Geometry check sheet. Reference: the model listing, model coordinates, mm. A direction names the side the tool comes from. Give positions to 0.01 mm unless a question says otherwise; leave off trailing zeros. Loops run counter-clockwise (first coordinate to the right, second up) from the corner with the lowest first, then second, coordinate; pieces in that order, holes last.
```python
from build123d import *

# Parameters (mm, degrees)
SKETCH1_R           = 1.35
BOSS_EXTRUDE1_DEPTH = 3
FILLET1_R           = 5
FILLET2_R           = 1
BOSS_EXTRUDE2_DEPTH = 7
BOSS_EXTRUDE3_DEPTH = 1
CUT_EXTRUDE1_REACH  = 74.282
SKETCH3_R           = 3
CIRPATTERN3_COUNT   = 3


with BuildPart() as part:
    # Sketch1 → Boss-Extrude1 (new body)
    with BuildSketch(Plane(origin=(0, 0, 0), x_dir=(1, 0, 0), z_dir=(0, 1, 0))):
        with BuildLine():
            ThreePointArc((-18.950510257, 23.9), (-22.286742625, 24.785806775), (-24.760474821, 22.378370572))
            Line((-24.760474821, 22.378370572), (-28.023324698, 24.262177826))
            Line((-28.023324698, 24.262177826), (-35.023324698, 12.137822174))
            Line((-35.023324698, 12.137822174), (-23.9, 5.715767665))
            Line((-23.9, 5.715767665), (-23.9, -18.950510257))
            ThreePointArc((-23.9, -18.950510257), (-23.874873734, -23.874873734), (-18.950510257, -23.9))
            Line((-18.950510257, -23.9), (-7, -23.9))
            Line((-7, -23.9), (-7, -36.4))
            Line((-7, -36.4), (7, -36.4))
            Line((7, -36.4), (7, -23.9))
            Line((7, -23.9), (18.950510257, -23.9))
            ThreePointArc((18.950510257, -23.9), (23.874873734, -23.874873734), (23.9, -18.950510257))
            Line((23.9, -18.950510257), (23.9, 5.715767665))
            Line((23.9, 5.715767665), (35.023324698, 12.137822174))
            Line((35.023324698, 12.137822174), (28.023324698, 24.262177826))
            Line((28.023324698, 24.262177826), (24.760474821, 22.378370572))
            ThreePointArc((24.760474821, 22.378370572), (22.286742625, 24.785806775), (18.950510257, 23.9))
            Line((18.950510257, 23.9), (-18.950510257, 23.9))
        make_face()
        with Locations(Location((-21.4, -21.4, 0), (0, 0, 270))):
            Circle(SKETCH1_R, mode=Mode.SUBTRACT)
        Polygon((15.364466094, -18.9), (-15.364466094, -18.9), (0, -3.535533906), align=None, mode=Mode.SUBTRACT)
        with Locations(Location((21.4, -21.4, 0), (0, 0, 270))):
            Circle(SKETCH1_R, mode=Mode.SUBTRACT)
        Polygon((-3.535533906, 0), (-18.9, -15.364466094), (-18.9, 15.364466094), align=None, mode=Mode.SUBTRACT)
        with Locations(Location((-21.4, 21.4, 0), (0, 0, 270))):
            Circle(SKETCH1_R, mode=Mode.SUBTRACT)
        Polygon((18.9, -15.364466094), (3.535533906, 0), (18.9, 15.364466094), align=None, mode=Mode.SUBTRACT)
        Polygon((0, 3.535533906), (-15.364466094, 18.9), (15.364466094, 18.9), align=None, mode=Mode.SUBTRACT)
        with Locations(Location((21.4, 21.4, 0), (0, 0, 270))):
            Circle(SKETCH1_R, mode=Mode.SUBTRACT)
    extrude(amount=BOSS_EXTRUDE1_DEPTH)

    # Fillet1
    # the kernel refuses this fillet: 5 mm, written as the material it adds along each edge
    with BuildSketch(Plane(origin=(7, 0, 23.9), x_dir=(0, 0, 1), z_dir=(0, 1, 0)), Plane(origin=(-7, 0, 23.9), x_dir=(-1, 0, 0), z_dir=(0, 1, 0))) as fillet1_piece_1:
        with BuildLine():
            CenterArc((FILLET1_R, FILLET1_R), FILLET1_R, 180, 90)
            Line((0, FILLET1_R), (-FILLET1_R * 0.02, FILLET1_R))
            Line((-FILLET1_R * 0.02, FILLET1_R), (-FILLET1_R * 0.02, -FILLET1_R * 0.02))
            Line((-FILLET1_R * 0.02, -FILLET1_R * 0.02), (FILLET1_R, -FILLET1_R * 0.02))
            Line((FILLET1_R, -FILLET1_R * 0.02), (FILLET1_R, 0))
        make_face()
    extrude(amount=3)
    with BuildSketch(Plane(origin=(23.9, 0, 18.950510257), x_dir=(0.5912237553807399, 0, 0.8065075765753815), z_dir=(0, 1, 0)), Plane(origin=(-18.950510257, 0, 23.9), x_dir=(-0.806507576575308, 0, 0.5912237553808403), z_dir=(0, 1, 0)), Plane(origin=(18.950510257, 0, -23.9), x_dir=(0.8065075765752107, 0, -0.591223755380973), z_dir=(0, 1, 0))) as fillet1_piece_2:
        with BuildLine():
            CenterArc((1.705620507, 4.94923638), FILLET1_R, 233.756102233, 28.072486936)
            Line((-1.25049827, 0.916698497), (-1.309620646, 0.836047739))
            Line((-1.309620646, 0.836047739), (-0.059122376, -0.080650758))
            Line((-0.059122376, -0.080650758), (0.014213504, -0.098984728))
            ThreePointArc((0.014213504, -0.098984728), (0.497472648, -0.064465466), (0.980731791, -0.098984728))
            Line((0.980731791, -0.098984728), (0.994945296, 0))
        make_face()
    extrude(amount=3)
    with BuildSketch(Plane(origin=(18.950510257, 0, 23.9), x_dir=(-1, 0, 0), z_dir=(0, 1, 0)), Plane(origin=(-23.9, 0, 18.950510257), x_dir=(0, 0, -1), z_dir=(0, 1, 0)), Plane(origin=(-18.950510257, 0, -23.9), x_dir=(1, 0, 0), z_dir=(0, 1, 0))) as fillet1_piece_3:
        with BuildLine():
            CenterArc((1.550510257, 5), FILLET1_R, 241.927513064, 28.072486936)
            Line((-0.802430919, 0.588235294), (-0.849489743, 0.5))
            ThreePointArc((-0.849489743, 0.5), (-0.439328974, 0.24212576), (-0.069985421, -0.071428571))
            Line((-0.069985421, -0.071428571), (0, -0.1))
            Line((0, -0.1), (1.550510257, -0.1))
            Line((1.550510257, -0.1), (1.550510257, 0))
        make_face()
    extrude(amount=3)
    with BuildSketch(Plane(origin=(-23.9, 0, -5.715767665), x_dir=(-0.8660254037844421, 0, -0.49999999999999417), z_dir=(0, 1, 0)), Plane(origin=(23.9, 0, -5.715767665), x_dir=(0, 0, 1), z_dir=(0, 1, 0))) as fillet1_piece_4:
        with BuildLine():
            CenterArc((FILLET1_R * 0.57735026919, FILLET1_R), FILLET1_R, 210, 60)
            Line((-FILLET1_R * 0.288675134595, FILLET1_R * 0.5), (-FILLET1_R * 0.30599564267, FILLET1_R * 0.49))
            Line((-FILLET1_R * 0.30599564267, FILLET1_R * 0.49), (-FILLET1_R * 0.0115470053838, -FILLET1_R * 0.02))
            Line((-FILLET1_R * 0.0115470053838, -FILLET1_R * 0.02), (FILLET1_R * 0.57735026919, -FILLET1_R * 0.02))
            Line((FILLET1_R * 0.57735026919, -FILLET1_R * 0.02), (FILLET1_R * 0.57735026919, 0))
        make_face()
    extrude(amount=3)
    with BuildSketch(Plane(origin=(24.760474821, 0, -22.378370572), x_dir=(-0.6125107821213894, 0, -0.7904622329909531), z_dir=(0, 1, 0))) as fillet1_piece_5:
        with BuildLine():
            CenterArc((4.405584254, -4.650844222), FILLET1_R, 111.538849964, 57.883583887)
            Line((-0.509452241, -3.733011854), (-0.607752971, -3.714655207))
            ThreePointArc((-0.607752971, -3.714655207), (-0.353807697, -1.852984049), (-0.099081577, 0.013521878))
            Line((-0.099081577, 0.013521878), (0.036713202, 0.093016884))
            ThreePointArc((0.036713202, 0.093016884), (1.284962074, -0.144409045), (2.533210946, 0.093016884))
            Line((2.533210946, 0.093016884), (2.569924148, 0))
        make_face()
    extrude(amount=3)
    with BuildSketch(Plane(origin=(-24.760474821, 0, -22.378370572), x_dir=(0.6125107821216187, 0, -0.7904622329907753), z_dir=(0, 1, 0))) as fillet1_piece_6:
        with BuildLine():
            CenterArc((4.405584254, 4.650844222), FILLET1_R, 190.577566149, 57.883583887)
            Line((-0.509452241, 3.733011854), (-0.607752971, 3.714655207))
            ThreePointArc((-0.607752971, 3.714655207), (-0.353807697, 1.852984049), (-0.099081577, -0.013521878))
            Line((-0.099081577, -0.013521878), (0.036713202, -0.093016884))
            ThreePointArc((0.036713202, -0.093016884), (1.284962074, 0.144409045), (2.533210946, -0.093016884))
            Line((2.533210946, -0.093016884), (2.569924148, 0))
        make_face()
    extrude(amount=3)

    # Fillet2
    fillet2_edges = [part.edges().sort_by_distance(p)[0] for p in [
        (15.364466094, 1.5, -18.9),
        (-15.364466094, 1.5, -18.9),
        (0, 1.5, -3.535533906),
        (-18.9, 1.5, 15.364466094),
        (-3.535533906, 1.5, 0),
        (-18.9, 1.5, -15.364466094),
        (18.9, 1.5, 15.364466094),
        (18.9, 1.5, -15.364466094),
        (3.535533906, 1.5, 0),
        (-15.364466094, 1.5, 18.9),
        (15.364466094, 1.5, 18.9),
        (0, 1.5, 3.535533906),
    ]]
    fillet(fillet2_edges, radius=FILLET2_R)

    # Sketch2 → Boss-Extrude2 (add, symmetric)
    with BuildSketch(Plane(origin=(0, 0, 0), x_dir=(0, 0, -1), z_dir=(1, 0, 0))):
        Polygon((-36.4, 3), (-36.4, 0), (-38.701980964, 0), (-44.462888601, 21.5), (-59.462888601, 21.5), (-59.462888601, 23), (-41.758983849, 23), align=None)
    boss_extrude2 = extrude(amount=BOSS_EXTRUDE2_DEPTH, both=True)

    # Sketch2<3> → Boss-Extrude3 (add, symmetric)
    with BuildSketch(Plane(origin=(0, 0, 0), x_dir=(0, 0, -1), z_dir=(1, 0, 0))):
        Polygon((-33.294171459, 3), (-36.4, 3), (-41.758983849, 23), (-38.653155307, 23), align=None)
    boss_extrude3 = extrude(amount=BOSS_EXTRUDE3_DEPTH, both=True)

    # Sketch3 → Cut-Extrude1 (cut, up to next)
    with BuildSketch(Plane.XZ.offset(-21.5), mode=Mode.PRIVATE) as cut_extrude1_sk1:
        with Locations(Location((0, 52.462888601, 0), (0, 0, 270))):
            Circle(SKETCH3_R)
    cut_extrude1_tool1 = extrude(cut_extrude1_sk1.sketch, amount=-CUT_EXTRUDE1_REACH, mode=Mode.PRIVATE) & part.part
    cut_extrude1 = cut_extrude1_tool1.solids().sort_by_distance((0, 21.5, 52.462889))[0]
    add(cut_extrude1, mode=Mode.SUBTRACT)

    # CirPattern3: Boss-Extrude2, Boss-Extrude3, Cut-Extrude1 ×3 about axis
    cirpattern3_axis = Axis((0, 0, 0), (0, 1, 0))
    add([boss_extrude2.rotate(cirpattern3_axis, i * 360 / CIRPATTERN3_COUNT) for i in range(1, CIRPATTERN3_COUNT)])
    add([boss_extrude3.rotate(cirpattern3_axis, i * 360 / CIRPATTERN3_COUNT) for i in range(1, CIRPATTERN3_COUNT)])
    add([cut_extrude1.rotate(cirpattern3_axis, i * 360 / CIRPATTERN3_COUNT) for i in range(1, CIRPATTERN3_COUNT)], mode=Mode.SUBTRACT)


solid = part.part
```
1) Sectioned sample at B-B on z = 21.4. Enter the section's corners in (x, y).
2) Sectioned sample at C-C on y = 16. Enter the section's corners in (x, z).
3) Mould release check, pull along X, two halves, no side actions. Record for faces 1 (the cylindrical face through (-42.46, 22.24, -25.84)), 2 (the flat face through (0.098, 10.6, 41.542)), 3 (the cylindrical face through (24.045, 1.479, 18.596)): +X half, -X half, draft (parallel to the pull), parting line (faces both ways), or undercut.
4) Sectioned sample at D-D on x = -46. Enter the section's corners in (y, z).
5) Tool access check on faces 4 (the flat face through (1, 13, 37)), 5 (the flat face through (-43, 21.5, -29)), 6 (the flat face through (31.95, 13.14, -19.6)), 7 (the flat face through (-32.785, 14.109, -27.011)), 8 (the flat face through (-18.9, 1, 0)). Record the directions out of +Z, -Z, +X, -X, +Y, -Y that give a thin tool (end or side, any length) a straight path to the whole face; none if there is none.
6) Sectioned sample at A-A on x = -21.4. Enter the section's corners in (y, z).
7) Depth check by flat-ended pin: P1, Ø1.5, axis at y = 2, z = 10, coming from the -X side; P2, Ø15.5, axis at x = -46.5, z = -26, coming from the -Y side; P3, Ø0.9, axis at x = 15.5, y = 1.5, coming from the +Z side. Enter the tip coordinate at first touch or a pass-through.
8) Scan lines: line 1 along X through (y, z) = (2.35, 21.4); line 2 along X through (y, z) = (0.8, -21.4); line 3 along X through (y, z) = (1.25, -16.5). Record each from-to range of solid material in increasing order.
Determined:
1. outline: (-24.9, 0) - (-22.75, 0) - (-22.75, 3) - (-24.9, 3) - close; (-20.05, 0) - (20.05, 0) - (20.05, 3) - (-20.05, 3) - close; (22.75, 0) - (24.9, 0) - (24.9, 3) - (22.75, 3) - close
2. outline: (-40.73, -15.43) - (-33.73, -27.56) - (-31.04, -26) - (-34.04, -20.81) - (-31.35, -19.25) - (-32.35, -17.52) - (-35.04, -19.08) - (-38.04, -13.88) - close; (-7, 39.88) - (-1, 39.88) - (-1, 36.78) - (1, 36.78) - (1, 39.88) - (7, 39.88) - (7, 42.99) - (-7, 42.99) - close; (31.04, -26) - (33.73, -27.56) - (40.73, -15.43) - (38.04, -13.88) - (35.04, -19.08) - (32.35, -17.52) - (31.35, -19.25) - (34.04, -20.81) - close
3. face 1: undercut
3. face 2: draft
3. face 3: +X half
4. outline: (21.5, -34.64) - (23, -34.64) - (23, -29.18) - (21.5, -29.18) - close; (21.5, -23.29) - (23, -23.29) - (23, -18.48) - (21.5, -18.48) - close
5. face 4: -Z, +X, +Y
5. face 5: -Z, -X, -Y
5. face 6: +Y
5. face 7: -Z, +Y, -Y
5. face 8: +Y, -Y
6. outline: (0, -24.9) - (3, -24.9) - (3, -22.75) - (0, -22.75) - close; (0, -20.05) - (3, -20.05) - (3, 20.05) - (0, 20.05) - close; (0, 22.75) - (3, 22.75) - (3, 24.9) - (0, 24.9) - close
7. P1: stops at x = -23.9
7. P2: stops at y = 21.5
7. P3: stops at z = 23.9
8. line 1: x = -24.9 to -22.75, -20.05 to 20.05, 22.75 to 24.9
8. line 2: x = -32.58 to -22.75, -20.05 to 20.05, 22.75 to 32.58
8. line 3: x = -35.55 to -12.96, 12.96 to 35.55
